Verification items for the finished model (mm, model axes). Round coordinates to 2 decimals unless told otherwise and drop trailing zeros. Write each loop counter-clockwise with the first axis right and the second up, starting at its lowest first coordinate (ties: lowest second). Pieces come first, ordered by that corner, then holes. Notation, with made-up numbers: (-8, -32) - (40, -32) arc R13 cw to (40, -18) - close; hole circle Ø5 at (0, 32). An arc over 180 degrees is marked (long way). Answer as a JSON object with one key per item and string values. Group by question number.
1) Thickness scan on line 1 (X direction, y = 10.5, z = -147.5); line 2 (Z direction, x = 151, y = 11.75); line 3 (X direction, y = 9.75, z = -37.5). Record the ranges inside material, lowest first.
2) Section check C-C (z = -256). Enter the section's corners in (x, y).
3) Section check A-A (y = 8.75). Enter the section's corners in (x, z).
4) Section check D-D (x = 617). Enter the section's corners in (y, z).
5) Section check B-B (x = 348.5). Enter the section's corners in (y, z), then the cut area to 3 significant figures.
6) Go/stop test with flat-tipped pins: pin 1 Ø1.9 at (x, y) = (173.5, 9.5) entering from -Z; pin 2 Ø1.9 at (y, z) = (9.5, -197.5) entering from +X; pin 3 Ø3 at (x, y) = (706.5, 8.5) entering from +Z; pin 4 Ø6 at (x, y) = (467, 2.5) entering from +Z. Record where each tip stops, or that it passes through.
```python
from build123d import *

# Parameters (mm, degrees)
SKETCH1_W           = 914.4
SKETCH1_H           = 304.8
BOSS_EXTRUDE1_DEPTH = 12.7
SKETCH2_W           = 914.4
SKETCH2_H           = 304.8
SKETCH2_W_2         = 304.8
SKETCH2_H_2         = 152.4
CUT_EXTRUDE1_DEPTH  = 6.35


with BuildPart() as part:
    # Sketch1 → Boss-Extrude1 (new body)
    with BuildSketch(Plane(origin=(0, 0, 0), x_dir=(1, 0, 0), z_dir=(0, 1, 0))):
        with Locations((457.2, 152.4)):
            Rectangle(SKETCH1_W, SKETCH1_H)
    extrude(amount=BOSS_EXTRUDE1_DEPTH)

    # Sketch2 → Cut-Extrude1 (cut)
    with BuildSketch(Plane(origin=(0, 12.7, 0), x_dir=(1, 0, 0), z_dir=(0, 1, 0))):
        with Locations((457.2, 152.4)):
            Rectangle(SKETCH2_W, SKETCH2_H)
        Polygon((330.2, 127), (12.7, 127), (12.7, 12.7), (901.7, 12.7), (901.7, 127), (584.2, 127), (584.2, 292.1), (330.2, 292.1), align=None, mode=Mode.SUBTRACT)
        with Locations((165.1, 215.9)):
            Rectangle(SKETCH2_W_2, SKETCH2_H_2, mode=Mode.SUBTRACT)
        with Locations((749.3, 215.9)):
            Rectangle(SKETCH2_W_2, SKETCH2_H_2, mode=Mode.SUBTRACT)
    extrude(amount=-CUT_EXTRUDE1_DEPTH, mode=Mode.SUBTRACT)


solid = part.part
```
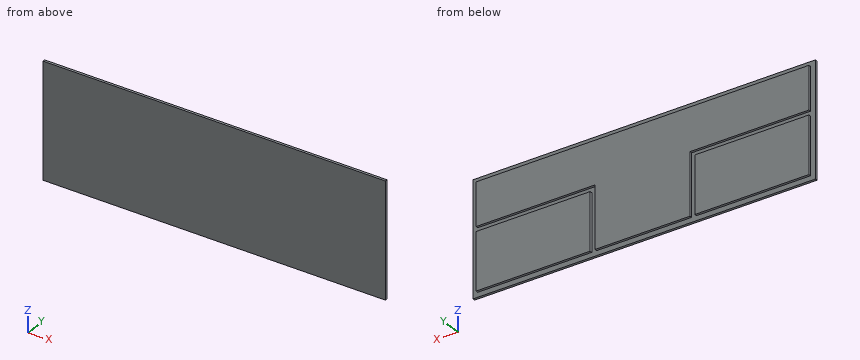
Returned:
{
 "1": {"line 1": "12.7 to 317.5, 330.2 to 584.2, 596.9 to 901.7", "line 2": "-292.1 to -139.7, -127 to -12.7", "line 3": "12.7 to 901.7"},
 "2": {"outline": "(0, 0) - (914.4, 0) - (914.4, 6.35) - (901.7, 6.35) - (901.7, 12.7) - (596.9, 12.7) - (596.9, 6.35) - (584.2, 6.35) - (584.2, 12.7) - (330.2, 12.7) - (330.2, 6.35) - (317.5, 6.35) - (317.5, 12.7) - (12.7, 12.7) - (12.7, 6.35) - (0, 6.35) - close"},
 "3": {"outline": "(12.7, -292.1) - (317.5, -292.1) - (317.5, -139.7) - (12.7, -139.7) - close; (12.7, -127) - (330.2, -127) - (330.2, -292.1) - (584.2, -292.1) - (584.2, -127) - (901.7, -127) - (901.7, -12.7) - (12.7, -12.7) - close; (596.9, -292.1) - (901.7, -292.1) - (901.7, -139.7) - (596.9, -139.7) - close"},
 "4": {"outline": "(0, -304.8) - (6.35, -304.8) - (6.35, -292.1) - (12.7, -292.1) - (12.7, -139.7) - (6.35, -139.7) - (6.35, -127) - (12.7, -127) - (12.7, -12.7) - (6.35, -12.7) - (6.35, 0) - (0, 0) - close"},
 "5": {"outline": "(0, -304.8) - (6.35, -304.8) - (6.35, -292.1) - (12.7, -292.1) - (12.7, -12.7) - (6.35, -12.7) - (6.35, 0) - (0, 0) - close", "area": "3,710 mm2"},
 "6": {"pin 1": "z = -292.1", "pin 2": "x = 901.7", "pin 3": "z = -12.7", "pin 4": "z = 0"}
}
